For this review, take the finished solid that the model builds, in its own axes (mm). Coordinates: 2 decimals unless noted, no trailing zeros. Order: outer loops, then holes, each group sorted by start corner. A loop starts at its lowest first (then second) coordinate and runs counter-clockwise, first axis right, second up.
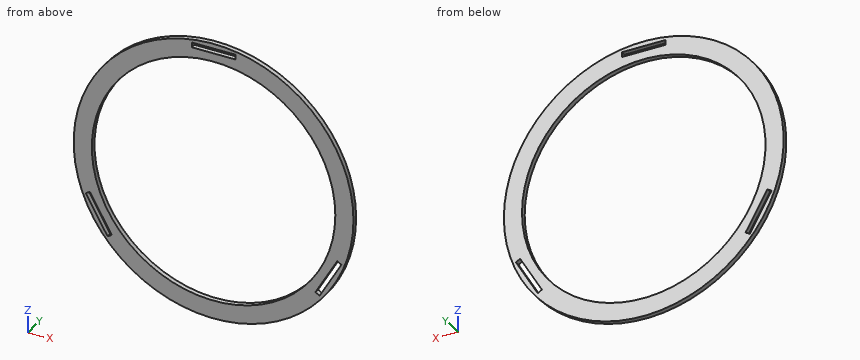
from build123d import *

# Parameters (mm, degrees)
SKETCH1_R           = 287.263450512
SKETCH1_R_2         = 250
BOSS_EXTRUDE1_DEPTH = 10
SKETCH2_W           = 89.558863324
SKETCH2_H           = 10
CUT_EXTRUDE1_DEPTH  = 10
CIRPATTERN1_COUNT   = 3


with BuildPart() as part:
    # Sketch1 → Boss-Extrude1 (new body)
    with BuildSketch(Plane(origin=(0, 0, 0), x_dir=(1, 0, 0), z_dir=(0, 1, 0))):
        Circle(SKETCH1_R)
        Circle(SKETCH1_R_2, mode=Mode.SUBTRACT)
    extrude(amount=BOSS_EXTRUDE1_DEPTH)

    # Sketch2 → Cut-Extrude1 (cut)
    with BuildSketch(Plane(origin=(0, 10, 0), x_dir=(1, 0, 0), z_dir=(0, 1, 0))):
        with Locations((0, -272.3)):
            Rectangle(SKETCH2_W, SKETCH2_H)
    cut_extrude1 = extrude(amount=-CUT_EXTRUDE1_DEPTH, mode=Mode.SUBTRACT)

    # CirPattern1: Cut-Extrude1 ×3 about axis
    cirpattern1_axis = Axis((0, 0, 0), (0, 1, 0))
    for i in range(1, CIRPATTERN1_COUNT):
        add(cut_extrude1.rotate(cirpattern1_axis, i * 360 / CIRPATTERN1_COUNT), mode=Mode.SUBTRACT)


solid = part.part
1. Take a section at B-B, the plane x = 0. Give the boundary of the cut face in (y, z).
Answer below:
outline: (0, -287.26) - (10, -287.26) - (10, -250) - (0, -250) - close; (0, 250) - (10, 250) - (10, 267.3) - (0, 267.3) - close; (0, 277.3) - (10, 277.3) - (10, 287.26) - (0, 287.26) - close
2. Take a section at D-D, the plane x = 169.5. Give the boundary of the cut face in (y, z).
Answer below:
outline: (0, -231.93) - (10, -231.93) - (10, -183.77) - (0, -183.77) - close; (0, 183.77) - (10, 183.77) - (10, 231.93) - (0, 231.93) - close
3. Clearance check with flat-ended pins moving along their axes: pin 1 Ø4 at (y, z) = (6.5, 194) entering from -X; pin 2 Ø3 at (y, z) = (7.5, -35.5) entering from -X; pin 3 Ø3 at (x, y) = (5, 2.5) entering from -Z. State where each tip first meets the part, or that it passes through.
Answer below:
pin 1: stops at x = -213.67
pin 2: stops at x = -285.24
pin 3: stops at z = -287.24
4. To check wall thickness, follow L1, parallel to Z at x = 0, y = 7.25; L2, parallel to X at y = 3, z = 0; L3, parallel to X at y = 3, z = 10. State the ranges of each line that lie inside material, in increasing order.
Answer below:
L1: z = -287.26 to -250, 250 to 267.3, 277.3 to 287.26
L2: x = -287.26 to -250, 250 to 287.26
L3: x = -287.09 to -249.8, 249.8 to 287.09
5. Take a section at C-C, the plane z = 0. Give the boundary of the cut face in (x, y), plus the area to 3 significant figures.
Answer below:
outline: (-287.26, 0) - (-250, 0) - (-250, 10) - (-287.26, 10) - close; (250, 0) - (287.26, 0) - (287.26, 10) - (250, 10) - close
area: 745 mm2
6. Take a section at A-A, the plane y = 3.75. Give the boundary of the cut face in (x, z), plus the area to 3 significant figures.
Answer below:
outline: circle Ø574.53 at (0, 0); hole (-262.54, -99.87) - (-217.76, -177.43) - (-209.1, -172.43) - (-253.88, -94.87) - close; hole circle Ø500 at (0, 0); hole (-44.78, 267.3) - (44.78, 267.3) - (44.78, 277.3) - (-44.78, 277.3) - close; hole (209.1, -172.43) - (217.76, -177.43) - (262.54, -99.87) - (253.88, -94.87) - close
area: 60,200 mm2
